from build123d import *

# Parameters (mm, degrees)
HELIX_CIRCLES_R     = 58.3
HELIX_CIRCLES_R_2   = 57
BOSS_EXTRUDE1_DEPTH = 103
SKETCH50_R          = 70.1085
BOSS_EXTRUDE2_DEPTH = 5.08
SKETCH58_R          = 70.104
SKETCH58_R_2        = 57
BOSS_EXTRUDE6_DEPTH = 5.08
SKETCH59_R          = 17.235790132
BOSS_EXTRUDE7_DEPTH = 7.62


with BuildPart() as part:
    # Helix_Circles → Boss-Extrude1 (new body)
    with BuildSketch(Plane(origin=(0, 0, 0), x_dir=(0, 0, -1), z_dir=(1, 0, 0))):
        Circle(HELIX_CIRCLES_R)
        Circle(HELIX_CIRCLES_R_2, mode=Mode.SUBTRACT)
    extrude(amount=BOSS_EXTRUDE1_DEPTH)

    # Sketch50 → Boss-Extrude2 (add)
    with BuildSketch(Plane(origin=(0, 0, 0), x_dir=(0, 0, -1), z_dir=(1, 0, 0))):
        Circle(SKETCH50_R)
    extrude(amount=-BOSS_EXTRUDE2_DEPTH)

    # Sketch58 → Boss-Extrude6 (add)
    with BuildSketch(Plane(origin=(103, 0, 0), x_dir=(0, 0, -1), z_dir=(1, 0, 0))):
        Circle(SKETCH58_R)
        Circle(SKETCH58_R_2, mode=Mode.SUBTRACT)
    extrude(amount=BOSS_EXTRUDE6_DEPTH)

    # Sketch59 → Boss-Extrude7 (add)
    with BuildSketch(Plane(origin=(0, 0, 0), x_dir=(0, 0, -1), z_dir=(1, 0, 0))):
        with Locations(Location((-25.38017448, 0, 0), (0, 0, 180))):
            Circle(SKETCH59_R)
        with Locations(Location((25.38017448, 0, 0), (0, 0, 180))):
            Circle(SKETCH59_R)
    extrude(amount=BOSS_EXTRUDE7_DEPTH)


solid = part.part
Source: CAD feature listing. Evaluate the final solid. Frame: model axes, mm. A direction names the side the tool comes from. Give positions to 0.01 mm unless a question says otherwise; leave off trailing zeros. Write each loop counter-clockwise with the first axis right and the second up, starting at its lowest first coordinate (ties: lowest second). Pieces come first, ordered by that corner, then holes. Notation, with made-up numbers: (69, 66) -> (118, 66) arc R26 cw to (118, 100) -> close; hole circle Ø3 at (-31, 52.5). An arc over 180 degrees is marked (long way). Return JSON: item names as keys, results as strings. Group by question number.
1. Section B-B, the plane y = 0. Output: boundary loops of the cut face in (x, z).
2. Access query for faces 1 (the face through (50.779, -56.914, 12.638)), 2 (the face through (0, 1, 1)), 3 (the face through (108.08, 57.4, 0.3)). Directions: +Z, -Z, +X, -X, +Y, -Y. A direction counts if a zero-diameter tool reaches every point of the face in a straight line with its end or side. Return the directions, or none.
3. Pin query (flat end, axial travel): pin 1 Ø4 at (x, z) = (88.5, 49) entering from -Y; pin 2 Ø2 at (y, z) = (31.5, 30) entering from +X; pin 3 Ø3 at (y, z) = (5.5, 38.5) entering from +X. Return the tip coordinate at first contact, or that it passes through.
4. Material intervals for line 1 (X direction, y = -30, z = 58); line 2 (Y direction, x = 41.5, z = 0); line 3 (Z direction, x = 43.5, y = -40.5), sorted ascending. Write a range as from..to.
5. Section C-C, the plane x = 74. Output: boundary loops of the cut face in (y, z).
6. Section A-A, the plane z = 0. Output: boundary loops of the cut face in (x, y), then the cut area to 3 significant figures.
7. Mould query, pull axis X, two halves, no side actions, for faces 4 (the face through (7.62, 0, 25)), 5 (the face through (3.76, -5.18, -8.94)), 6 (the face through (0, 10.7, 57.5)). Classes: +X half, -X half, draft (parallel to the pull), parting line (faces both ways), or undercut.
8. Section D-D, the plane z = 45. Output: boundary loops of the cut face in (x, y).
Determined:
{
 "1": {"outline": "(-5.08, -70.11) -> (0, -70.11) -> (0, -58.3) -> (103, -58.3) -> (103, -70.1) -> (108.08, -70.1) -> (108.08, -57) -> (0, -57) -> (0, -42.62) -> (7.62, -42.62) -> (7.62, -8.14) -> (0, -8.14) -> (0, 8.14) -> (7.62, 8.14) -> (7.62, 42.62) -> (0, 42.62) -> (0, 57) -> (108.08, 57) -> (108.08, 70.1) -> (103, 70.1) -> (103, 58.3) -> (0, 58.3) -> (0, 70.11) -> (-5.08, 70.11) -> close"},
 "2": {"face 1": "none", "face 2": "+X", "face 3": "+Z, -Z, +X, +Y, -Y"},
 "3": {"pin 1": "stops at y = -34.49", "pin 2": "stops at x = 0", "pin 3": "stops at x = 7.62"},
 "4": {"line 1": "x = -5.08..0, 103..108.08", "line 2": "y = -58.3..-57, 57..58.3", "line 3": "z = -41.94..-40.11, 40.11..41.94"},
 "5": {"outline": "circle Ø116.6 at (0, 0); hole circle Ø114 at (0, 0)"},
 "6": {"outline": "(-5.08, -70.11) -> (0, -70.11) -> (0, -58.3) -> (103, -58.3) -> (103, -70.1) -> (108.08, -70.1) -> (108.08, -57) -> (0, -57) -> (0, 57) -> (108.08, 57) -> (108.08, 70.1) -> (103, 70.1) -> (103, 58.3) -> (0, 58.3) -> (0, 70.11) -> (-5.08, 70.11) -> close", "area": "1,110 mm2"},
 "7": {"face 4": "+X half", "face 5": "draft", "face 6": "undercut"},
 "8": {"outline": "(-5.08, -53.76) -> (0, -53.76) -> (0, -37.07) -> (103, -37.07) -> (103, -53.75) -> (108.08, -53.75) -> (108.08, -34.99) -> (0, -34.99) -> (0, 34.99) -> (108.08, 34.99) -> (108.08, 53.75) -> (103, 53.75) -> (103, 37.07) -> (0, 37.07) -> (0, 53.76) -> (-5.08, 53.76) -> close"}
}
